The model under review builds one solid part; all positions refer to its coordinate system, in mm. Face numbers are marked on the shaded views. Round coordinates to 2 decimals unless told otherwise and drop trailing zeros. Answer as CSV lines item,"result".
from build123d import *

# Parameters (mm, degrees)
F0_R          = 9.525
F0_R_2        = 6.35
F1_DEPTH      = 25.4
F3_DEPTH      = 25.4
F3_DEPTH_BACK = 25.4
F4_R          = 1.27
F5_T          = -2.54


with BuildPart() as f1:
    # F0 (on Top) → F1 (new body)
    with BuildSketch(Plane.XY):
        with BuildLine():
            ThreePointArc((1.6565217391, 12.5915025207), (9.5479795268, 8.3741320121), (12.7, 0))
            ThreePointArc((12.7, 0), (10.1185149246, -7.6750020013), (3.4235187843, -12.229861779))
            Line((3.4235187843, -12.229861779), (37.5185084512, -7.8734905376))
            ThreePointArc((37.5185084512, -7.8734905376), (28.5750137634, 0.0147815331), (37.547826087, 7.8696890754))
            Line((37.547826087, 7.8696890754), (1.6565217391, 12.5915025207))
        make_face()
        with BuildLine():
            ThreePointArc((3.4235187843, -12.229861779), (10.1185149246, -7.6750020013), (12.7, 0))
            ThreePointArc((12.7, 0), (9.5479795268, 8.3741320121), (1.6565217391, 12.5915025207))
            ThreePointArc((1.6565217391, 12.5915025207), (-12.6679412042, -0.9018124228), (3.4235187843, -12.229861779))
        make_face()
        Circle(F0_R, mode=Mode.SUBTRACT)
        with BuildLine():
            ThreePointArc((44.45, 0), (42.4799872042, 5.2338325076), (37.547826087, 7.8696890754))
            ThreePointArc((37.547826087, 7.8696890754), (28.5750137634, 0.0147815331), (37.5185084512, -7.8734905376))
            ThreePointArc((37.5185084512, -7.8734905376), (42.4702302025, -5.244936328), (44.45, 0))
        make_face()
        with Locations((36.5125, 0)):
            Circle(F0_R_2, mode=Mode.SUBTRACT)
    extrude(amount=F1_DEPTH)

    # F2 (on Front) → F3 (cut, two sides)
    with BuildSketch(Plane.XZ) as f3_sk:
        Polygon((44.45, 10.4004494442), (15.875, 0), (44.45, 0), align=None)
    extrude(amount=-F3_DEPTH, mode=Mode.SUBTRACT)
    extrude(f3_sk.sketch, amount=F3_DEPTH_BACK, mode=Mode.SUBTRACT)

    # F4
    f4_edges = [f1.edges().sort_by_distance(p)[0] for p in [
        (26.711413, 9.295314, 3.944132),
        (-12.667941, -0.901812, 0),
        (8.765761, 11.65622, 0),
        (9.649259, -11.434389, 0),
        (15.875, 0.041011, 0),
    ]]
    fillet(f4_edges, radius=F4_R)

    # F5
    f5_openings = [f1.faces().sort_by_distance(p)[0] for p in [
        (15.37002, 0.035477, 25.4),
    ]]
    offset(amount=F5_T, openings=f5_openings)


solid = f1.part
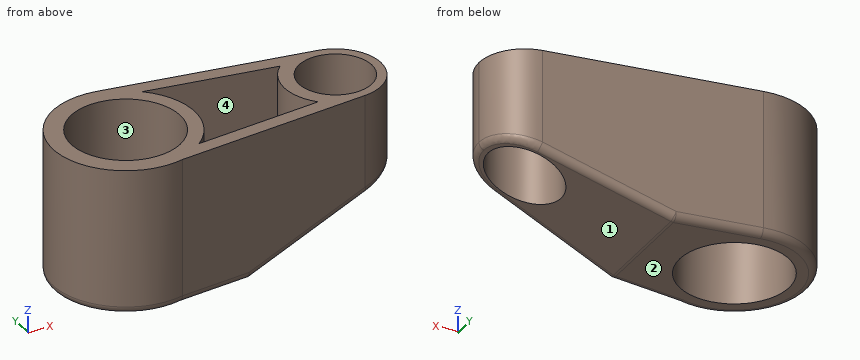
1. Wall thickness on probe 1 along X at (y, z) = (0.25, 17.5); probe 2 along Y at (x, z) = (0, 18.5) (3 decimals); probe 3 along X at (y, z) = (1.25, 10.5): over which ranges is each line inside the solid? List them lowest first.
Numbers:
probe 1,"x = -12.7 to -9.52, 9.52 to 12.06, 27.63 to 30.17, 42.86 to 44.45"
probe 2,"y = -12.7 to -9.525, 9.525 to 12.7"
probe 3,"x = -12.64 to -9.44, 9.44 to 12, 27.71 to 30.29, 42.74 to 44.1"
2. Take a section at A-A (z = 23.75). State how many separate pieces and enclosed holes the cut face has, plus the area to 3 significant figures.
Numbers:
separate pieces,"1"
enclosed holes,"3"
area,"429 mm²"
3. Clearance check with flat-ended pins moving along their axes: pin 1 (2 mm diameter, centred on x = 37.5, z = 6, fed in from +Y); pin 2 (3 mm diameter, centred on x = 23, y = -6, fed in from +Z); pin 3 (2 mm diameter, centred on y = 0, z = 9.5, fed in from +X). State where each tip first meets the part, or that it passes through.
Numbers:
pin 1,"passes through"
pin 2,"stops at z = 25.4"
pin 3,"stops at x = 44.17"
4. Draft analysis for pull direction X (two halves, no side actions). For the marked faces 1, 2, 3 and 4, state which applies: +X half, -X half, draft (parallel to the pull), parting line (faces both ways), or undercut.
Numbers:
face 1,"+X half"
face 2,"draft"
face 3,"undercut"
face 4,"undercut"
